Here's how the part is built. I have some questions about the finished solid (model axes, mm). A direction names the side the tool comes from. Coordinates: 2 decimals unless noted, no trailing zeros. Write each loop counter-clockwise with the first axis right and the second up, starting at its lowest first coordinate (ties: lowest second). Pieces come first, ordered by that corner, then holes. Notation, with made-up numbers: (74.5, 49.5) -> (118.5, 49.5) arc R20 ccw to (118.5, 71.5) -> close; hole circle Ø6 at (12, 80). An arc over 180 degrees is marked (long way). Put each result on its own line as item: value.
```python
from build123d import *

# Parameters (mm, degrees)
F0_W     = 50.8
F0_H     = 50.8
F0_R     = 21.309013
F1_DEPTH = 25.4
F2_DEPTH = 22.86
F3_DEPTH = 24.13


with BuildPart() as f1:
    # F0 (on Front) → F1 (new body)
    with BuildSketch(Plane.XZ):
        with Locations((25.4, 25.4)):
            Rectangle(F0_W, F0_H)
        with Locations((25.4, 25.4)):
            Circle(F0_R, mode=Mode.SUBTRACT)
    extrude(amount=F1_DEPTH)

    # F0 (on Front) → F2 (join)
    with BuildSketch(Plane.XZ):
        with Locations((25.4, 25.4)):
            Circle(F0_R)
        Polygon((13.571316, 14.178988), (25.4, 42.942073), (37.675597, 14.178988), align=None, mode=Mode.SUBTRACT)
    extrude(amount=F2_DEPTH)

    # F0 (on Front) → F3 (join)
    with BuildSketch(Plane.XZ):
        Polygon((37.675597, 14.178988), (25.4, 42.942073), (13.571316, 14.178988), align=None)
    extrude(amount=F3_DEPTH)


solid = f1.part
```
Item 1: Imagine slicing it at A-A on x = 19. Write out the boundary of the cut face in (y, z).
Output:
outline: (-25.4, 0) -> (0, 0) -> (0, 50.8) -> (-25.4, 50.8) -> (-25.4, 45.73) -> (-22.86, 45.73) -> (-22.86, 27.38) -> (-24.13, 27.38) -> (-24.13, 14.18) -> (-22.86, 14.18) -> (-22.86, 5.07) -> (-25.4, 5.07) -> close
Item 2: Which directions (+Z, -Z, +X, -X, +Y, -Y) give clear straight access to the entire face, cutting with the end or side of a thin tool? Please do faces 4 (the flat face through (50.8, -13, 25)), 5 (the cylindrical face through (45.725, -24.112, 31.801)).
Output:
face 4: +Z, -Z, +X, +Y, -Y
face 5: -Y
Item 3: For P1, Ø1, axis at x = 37.5, z = 22.5, coming from the -Y side; P2, Ø4, axis at x = 24, z = 40, coming from the +Y side; P3, Ø13, axis at x = 32.5, z = 27, coming from the -Y side, each with a flat end and sliding along its axis, tell me the tip position at first contact or that it passes through.
Output:
P1: stops at y = -22.86
P2: stops at y = 0
P3: stops at y = -24.13
Item 4: If we mould it in two halves opening along Z, with no side actions, what happens to faces 1 (the flat face through (31.624, -23.486, 28.359)), 2 (the flat face through (0, -13, 25)), 3 (the flat face through (25, -13, 50.8))? For each: released by +Z, released by -Z, zero draft, split by the parting line, or undercut.
Output:
face 1: undercut
face 2: zero draft
face 3: released by +Z
Item 5: Please list where these lines run through material, in increasing order: line 1 along Z through (x, y) = (25.4, -24.5); line 2 along X through (y, z) = (-24, 23.5); line 3 along Y through (x, z) = (38.5, 40). Write a range as from..to.
Output:
line 1: z = 0..4.09, 46.71..50.8
line 2: x = 0..4.18, 17.4..33.7, 46.62..50.8
line 3: y = -22.86..0
Item 6: Imagine slicing it at C-C on z = 8.5. Write out the boundary of the cut face in (x, y).
Output:
outline: (0, -25.4) -> (12.42, -25.4) -> (12.42, -22.86) -> (38.38, -22.86) -> (38.38, -25.4) -> (50.8, -25.4) -> (50.8, 0) -> (0, 0) -> close
Item 7: Imagine slicing it at B-B on z = 39. Write out the boundary of the cut face in (x, y), then the cut area to 3 significant figures.
Output:
outline: (0, -25.4) -> (9, -25.4) -> (9, -22.86) -> (23.78, -22.86) -> (23.78, -24.13) -> (27.08, -24.13) -> (27.08, -22.86) -> (41.8, -22.86) -> (41.8, -25.4) -> (50.8, -25.4) -> (50.8, 0) -> (0, 0) -> close
area: 1,210 mm²
